The drawing under review shows one solid part. Ordinate dimensions are in mm from its lowest x, y, z. Coordinates: 2 decimals unless noted, no trailing zeros. Write each loop counter-clockwise with the first axis right and the second up, starting at its lowest first coordinate (ties: lowest second). Pieces come first, ordered by that corner, then holes.
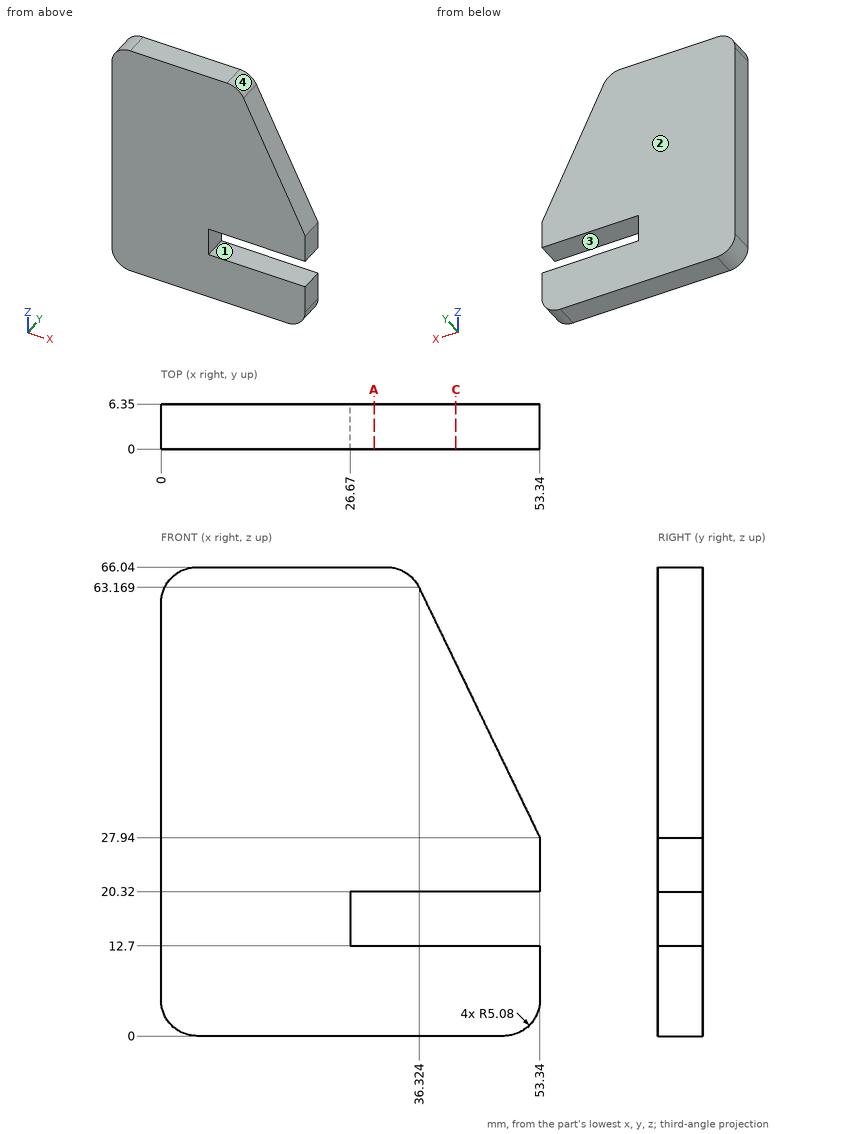
1) Clearance check with flat-ended pins moving along their axes: P1, Ø12, axis at x = 19.5, z = 28, coming from the -Y side; P2, Ø3, axis at x = 42.5, y = 4, coming from the +Z side; P3, Ø3, axis at x = 48, y = 2, coming from the +Z side. State where each tip first meets the part, or that it passes through.
2) Consider section A-A (x = 30). Give the boundary of the cut face in (y, z).
3) The part is to be moulded in two halves that separate along Z. For the marked faces 1, 2, 3 and 4, say which applies: pulls with the +Z half, pulls with the -Z half, needs draft (parallel to the pull), parting line crosses it, or undercut.
4) Consider section C-C (x = 41.5). Give the boundary of the cut face in (y, z), then the cut area to 3 significant figures.
5) For L1, parallel to Z at x = 30, y = 6; L2, parallel to Z at x = 34, y = 5 (1 decimal); L3, parallel to X at y = 5.5, z = 28, list the stretches that pass through material, from the lowest coordinate up.
Results:
1. P1: stops at y = 0
1. P2: stops at z = 53.49
1. P3: stops at z = 42.1
2. outline: (0, 0) - (6.35, 0) - (6.35, 12.7) - (0, 12.7) - close; (0, 20.32) - (6.35, 20.32) - (6.35, 66.04) - (0, 66.04) - close
3. face 1: undercut
3. face 2: needs draft
3. face 3: undercut
3. face 4: pulls with the +Z half
4. outline: (0, 0) - (6.35, 0) - (6.35, 12.7) - (0, 12.7) - close; (0, 20.32) - (6.35, 20.32) - (6.35, 52.45) - (0, 52.45) - close
4. area: 285 mm2
5. L1: z = 0 to 12.7, 20.32 to 66.04
5. L2: z = 0 to 12.7, 20.3 to 65.5
5. L3: x = 0 to 53.31
